from build123d import *

# Parameters (mm, degrees)
F3_DEPTH      = 25
F6_DEPTH      = 25
F6_DEPTH_BACK = 25
F8_DEPTH      = 25
F8_DEPTH_BACK = 25
F10_R         = 24
F11_DEPTH     = 6
F13_DEPTH     = 1
F15_R         = 23.5
F16_DEPTH     = 1.5
F17_R         = 1
F18_R         = 20
F19_DEPTH     = 2
F19_TAPER     = 35
F20_R         = 21
F21_DEPTH     = 1


# Not quite as in the source:
# - a fillet or chamfer that OpenCascade refuses, or shapes differently, is made with other operations: its cross-section is extruded or revolved along the edge and cut away or added


with BuildPart() as f3:
    # F2 (on Top) → F3 (new body)
    with BuildSketch(Plane.XY):
        with BuildLine():
            Line((-13, 20.1742410018), (-13, 26.1742410018))
            Line((-13, 26.1742410018), (-15.6435015354, 26.1742410018))
            ThreePointArc((-15.6435015354, 26.1742410018), (-17.78469231, 18.672379989), (-21.0241029415, 11.5752795))
            ThreePointArc((-21.0241029415, 11.5752795), (-17.5469493067, 16.3738990478), (-13, 20.1742410018))
        make_face()
    extrude(amount=F3_DEPTH)


with BuildPart() as f3b:
    # F2 (on Top) → F3, piece 2 (new body)
    with BuildSketch(Plane.XY):
        with BuildLine():
            Line((13, 26.1742410018), (13, 20.1742410018))
            ThreePointArc((13, 20.1742410018), (17.5469493067, 16.3738990478), (21.0241029415, 11.5752795))
            ThreePointArc((21.0241029415, 11.5752795), (17.78469231, 18.672379989), (15.6435015354, 26.1742410018))
            Line((15.6435015354, 26.1742410018), (13, 26.1742410018))
        make_face()
    extrude(amount=F3_DEPTH)


with BuildPart() as f3c:
    # F2 (on Top) → F3, piece 3 (new body)
    with BuildSketch(Plane.XY):
        with BuildLine():
            ThreePointArc((-13, -20.1742410018), (-17.5469493067, -16.3738990478), (-21.0241029415, -11.5752795))
            ThreePointArc((-21.0241029415, -11.5752795), (-17.78469231, -18.672379989), (-15.6435015354, -26.1742410018))
            Line((-15.6435015354, -26.1742410018), (-13, -26.1742410018))
            Line((-13, -26.1742410018), (-13, -20.1742410018))
        make_face()
    extrude(amount=F3_DEPTH)


with BuildPart() as f3d:
    # F2 (on Top) → F3, piece 4 (new body)
    with BuildSketch(Plane.XY):
        with BuildLine():
            ThreePointArc((15.6435015354, -26.1742410018), (17.78469231, -18.672379989), (21.0241029415, -11.5752795))
            ThreePointArc((21.0241029415, -11.5752795), (17.5469493067, -16.3738990478), (13, -20.1742410018))
            Line((13, -20.1742410018), (13, -26.1742410018))
            Line((13, -26.1742410018), (15.6435015354, -26.1742410018))
        make_face()
    extrude(amount=F3_DEPTH)


with BuildPart() as f6_tool:
    # F5 (on Right) → F6 (new body, two sides)
    with BuildSketch(Plane.YZ) as f6_sk:
        with BuildLine():
            Line((23.5471649475, 7.1683851421), (27.7989016838, 1.9778330012))
            Line((27.7989016838, 1.9778330012), (27.7989016838, 26.740285454))
            Line((27.7989016838, 26.740285454), (-29.0615007661, 26.740285454))
            Line((-29.0615007661, 26.740285454), (-27.7989016838, 1.9778330012))
            Line((-27.7989016838, 1.9778330012), (-23.5471649475, 7.1683851421))
            ThreePointArc((-23.5471649475, 7.1683851421), (-21.8190448857, 8.5189558788), (-19.6791764535, 8.999999905))
            Line((-19.6791764535, 8.999999905), (0, 8.999999905))
            Line((0, 8.999999905), (19.6791764535, 8.999999905))
            ThreePointArc((19.6791764535, 8.999999905), (21.8190448857, 8.5189558788), (23.5471649475, 7.1683851421))
        make_face()
    extrude(amount=-F6_DEPTH)
    extrude(f6_sk.sketch, amount=F6_DEPTH_BACK)


with BuildPart() as f3_1:
    add(f3.part)

    # F6: cut by f6_tool
    add(f6_tool.part, mode=Mode.SUBTRACT)


with BuildPart() as f3b_1:
    add(f3b.part)

    # F6: cut by f6_tool
    add(f6_tool.part, mode=Mode.SUBTRACT)


with BuildPart() as f3c_1:
    add(f3c.part)

    # F6: cut by f6_tool
    add(f6_tool.part, mode=Mode.SUBTRACT)


with BuildPart() as f3d_1:
    add(f3d.part)

    # F6: cut by f6_tool
    add(f6_tool.part, mode=Mode.SUBTRACT)


with BuildPart() as f8_tool:
    # F7 (on Right) → F8 (new body, two sides)
    with BuildSketch(Plane.YZ) as f8_sk:
        with BuildLine():
            Line((17.8908835105, 3), (0, 3))
            Line((0, 3), (-17.8908835105, 3))
            ThreePointArc((-17.8908835105, 3), (-19.7544863974, 2.639718125), (-21.3495203475, 1.6107937119))
            Line((-21.3495203475, 1.6107937119), (-22.0408191574, 0.9486258563))
            ThreePointArc((-22.0408191574, 0.9486258563), (-22.6937657116, 0.6715368573), (-23.3662235722, 0.8971868999))
            Line((-23.3662235722, 0.8971868999), (-25.727452218, 2.8313400119))
            ThreePointArc((-25.727452218, 2.8313400119), (-26.1117766069, 3.5541907786), (-25.8675033398, 4.3355671527))
            Line((-25.8675033398, 4.3355671527), (-26.6892556101, 5.8121909387))
            Line((-26.6892556101, 5.8121909387), (-28.4930374473, 3.2282707538))
            Line((-28.4930374473, 3.2282707538), (-28.1138848513, -2.6890258305))
            Line((-28.1138848513, -2.6890258305), (27.818409726, -2.2570919245))
            Line((27.818409726, -2.2570919245), (26.8063536115, 3.2282707538))
            Line((26.8063536115, 3.2282707538), (26.1989608407, 4.4945557602))
            Line((26.1989608407, 4.4945557602), (25.8675033398, 4.3355671527))
            ThreePointArc((25.8675033398, 4.3355671527), (26.1117766069, 3.5541907786), (25.727452218, 2.8313400119))
            Line((25.727452218, 2.8313400119), (23.3662235722, 0.8971868999))
            ThreePointArc((23.3662235722, 0.8971868999), (22.6937657116, 0.6715368573), (22.0408191574, 0.9486258563))
            Line((22.0408191574, 0.9486258563), (21.3495203475, 1.6107937119))
            ThreePointArc((21.3495203475, 1.6107937119), (19.7544863974, 2.639718125), (17.8908835105, 3))
        make_face()
    extrude(amount=-F8_DEPTH)
    extrude(f8_sk.sketch, amount=F8_DEPTH_BACK)


with BuildPart() as f3_2:
    add(f3_1.part)

    # F8: cut by f8_tool
    add(f8_tool.part, mode=Mode.SUBTRACT)



with BuildPart() as f3b_2:
    add(f3b_1.part)

    # F8: cut by f8_tool
    add(f8_tool.part, mode=Mode.SUBTRACT)


with BuildPart() as f3c_2:
    add(f3c_1.part)

    # F8: cut by f8_tool
    add(f8_tool.part, mode=Mode.SUBTRACT)


with BuildPart() as f3d_2:
    add(f3d_1.part)

    # F8: cut by f8_tool
    add(f8_tool.part, mode=Mode.SUBTRACT)


with BuildPart() as f3_3:
    add(f3_2.part)

    add(f3b_2.part)  # F11 merges F3b

    add(f3c_2.part)  # F11 merges F3c

    add(f3d_2.part)  # F11 merges F3d
    # F10 (on plane+point) → F11 (join)
    with BuildSketch(Plane.XY.offset(3)):
        Circle(F10_R)
    extrude(amount=F11_DEPTH)

    # F12 (on face) → F13 (join)
    with BuildSketch(Plane(origin=(0, 0, 3), x_dir=(1, 0, 0), z_dir=(0, 0, -1))):
        with BuildLine():
            ThreePointArc((23, 0), (16.2634559673, 16.2634559673), (0, 23))
            ThreePointArc((0, 23), (-16.2634559673, 16.2634559673), (-23, 0))
            ThreePointArc((-23, 0), (-16.2634559673, -16.2634559673), (0, -23))
            ThreePointArc((0, -23), (16.2634559673, -16.2634559673), (23, 0))
        make_face()
    extrude(amount=F13_DEPTH)

    # F14: fillet of radius 5 on 1 edges, made by hand

    # F14_s1 → F14_t2 (revolve, cut)
    with BuildSketch(Plane.YZ):
        with BuildLine():
            ThreePointArc((23, 3), (21.5811388301, 2.2565835097), (20, 2))
            Line((20, 2), (23, 2))
            Line((23, 2), (23, 3))
        make_face()
    revolve(axis=Axis((0, 0, 2), (0, 0, 1)), mode=Mode.SUBTRACT)

    # F15 (on face) → F16 (join)
    with BuildSketch(Plane.XY.offset(8.999999905)):
        Circle(F15_R)
    extrude(amount=F16_DEPTH)

    # F17
    f17_edges = [f3_3.edges().sort_by_distance(p)[0] for p in [
        (-23.5, 0, 10.5),
    ]]
    fillet(f17_edges, radius=F17_R)

    # F18 (on face) → F19 (cut)
    with BuildSketch(Plane.XY.offset(10.499999905)):
        Circle(F18_R)
    extrude(amount=-F19_DEPTH, taper=F19_TAPER, mode=Mode.SUBTRACT)

    # F20 (on face) → F21 (cut)
    with BuildSketch(Plane.XY.offset(10.499999905)):
        with Locations((0.4080029248, 0)):
            Circle(F20_R)
    extrude(amount=-F21_DEPTH, mode=Mode.SUBTRACT)


solid = f3_3.part
Design review of the part built by this model. Coordinates are the model's own, in mm. A direction names the side the tool comes from. Coordinates: 2 decimals unless noted, no trailing zeros. Loops run counter-clockwise (first coordinate to the right, second up) from the corner with the lowest first, then second, coordinate; pieces in that order, holes last. Notation, with made-up numbers: M 83,44.25 L 140,44.25 A25 ccw 140,63.25 Z; hole C -8.75,84.5 d5. An arc over 180 degrees is marked long. Answer as CSV lines item,"result".
Item 1: For P1, Ø12, axis at x = 0.5, y = 3.5, coming from the -Z side; P2, Ø3, axis at y = 22, z = 6, coming from the -X side; P3, Ø1, axis at x = 11, z = 4.5, coming from the +Y side, all flat-tipped, find the tip position at first contact; note any pin that passes through.
Answer list:
P1,"z = 2"
P2,"x = -17.15"
P3,"y = 21.58"
Item 2: For probe 1 along Z at (x, y) = (12.5, -10); probe 2 along Y at (x, z) = (-0.5, 8.75); probe 3 along Z at (x, y) = (2, -21.5), list the stretches that pass through material, from the lowest coordinate up.
Answer list:
probe 1,"2 to 8.5"
probe 2,"-23.99 to -18.77, 18.77 to 23.99"
probe 3,"2.26 to 10.5"
Item 3: Machinability: for faces 1 (the face through (-14.651, 24.691, 5.772)), 2 (the face through (-15.58, -19.73, 2.65)), 3 (the face through (14.69, -21.847, 8.506)), which of the approach directions +Z, -Z, +X, -X, +Y, -Y give a long, thin tool a straight path to every point of the face, cutting with its end or side? Answer none if there is none.
Answer list:
face 1,"+Z, -X, +Y"
face 2,"-Z, -X"
face 3,"+Z, +X, -Y"
Item 4: Add section A-A on z = 7.75. State the section outline as (x, y) points.
Answer list:
outline,"M -21.02,-11.58 A52 cw -16.4,-22.99 L -13,-22.99 L -13,-20.17 A24 ccw 13,-20.17 L 13,-22.99 L 16.4,-22.99 A52 cw 21.02,-11.58 A24 ccw 21.02,11.58 A52 cw 16.4,22.99 L 13,22.99 L 13,20.17 A24 ccw -13,20.17 L -13,22.99 L -16.4,22.99 A52 cw -21.02,11.58 A24 ccw Z"
Item 5: Add section B-B on x = 0. State the section outline as (y, z) points.
Answer list:
outline,"M -24,3 L -23,3 A5 ccw -20,2 L 20,2 A5 ccw 23,3 L 24,3 L 24,9 L 23.5,9 L 23.5,9.5 A1 ccw 22.5,10.5 L 21,10.5 L 21,9.5 L 19.3,9.5 L 18.6,8.5 L -18.6,8.5 L -19.3,9.5 L -21,9.5 L -21,10.5 L -22.5,10.5 A1 ccw -23.5,9.5 L -23.5,9 L -24,9 Z"
Item 6: The part is to be moulded in two halves that separate along X. For faces 4 (the face through (22.4, 7.1, 9.2)), 5 (the face through (0, -24, 6)), 6 (the face through (24, 0, 6)), say which applies: pulls with the +X half, pulls with the -X half, needs draft (parallel to the pull), parting line crosses it, or undercut.
Answer list:
face 4,"parting line crosses it"
face 5,"undercut"
face 6,"pulls with the +X half"
